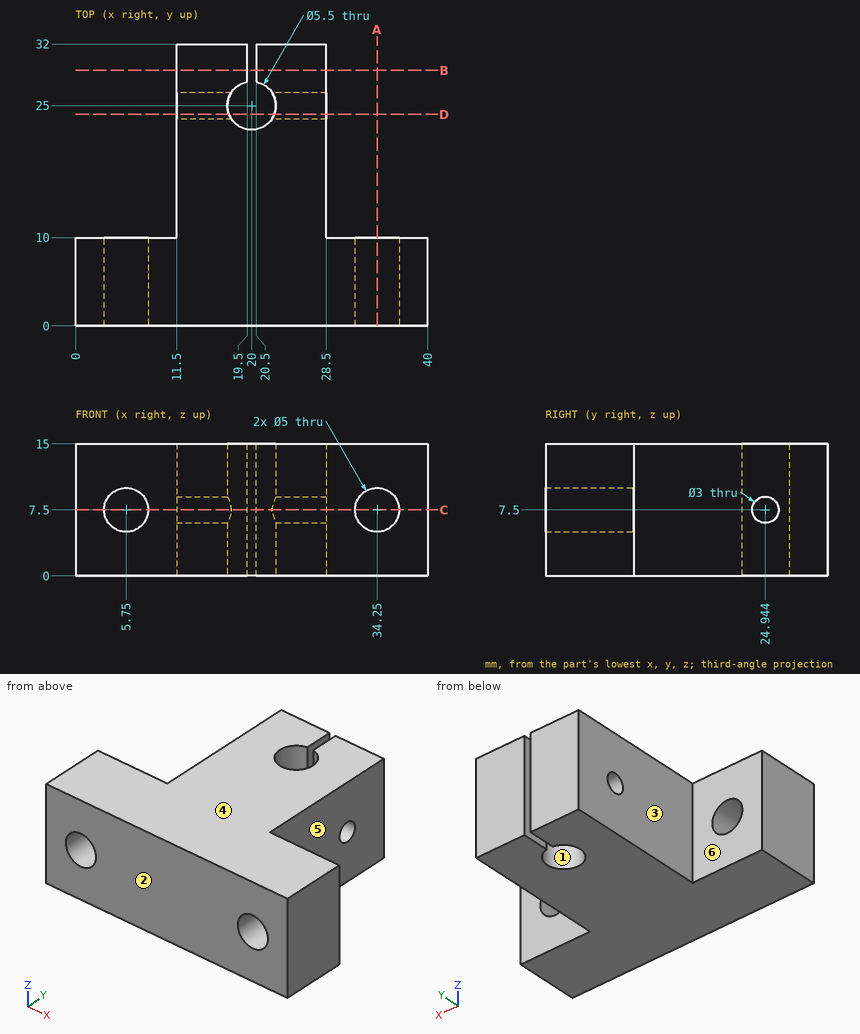
Could you check a few things on this drawing? It's one solid part, dimensions in mm from its lowest x, y, z. A direction names the side the tool comes from. Coordinates: 2 decimals unless noted, no trailing zeros. Loops run counter-clockwise (first coordinate to the right, second up) from the corner with the lowest first, then second, coordinate; pieces in that order, holes last.
1. Imagine slicing it at C-C (z = 7.5). Please give me the cut outline in (x, y).
2. Imagine slicing it at A-A (x = 34.25). Please give me the cut outline in (y, z), and give its area (3 significant figures).
3. Imagine slicing it at D-D (y = 24). Please give me the cut outline in (x, z).
4. For P1, Ø4.5, axis at x = 34.25, z = 7.5, coming from the -Y side; P2, Ø2, axis at y = 29.5, z = 7, coming from the -X side; P3, Ø4.5, axis at y = 29, z = 9, coming from the +X side; P4, Ø6, axis at x = 3.5, z = 11, coming from the +Y side, each with a flat end and sliding along its axis, tell me the tip position at first contact or that it passes through.
5. I need wall thicknesses on L1, parallel to X at y = 25, z = 13; L2, parallel to Z at x = 34.25, y = 2.75; L3, parallel to X at y = 30.5, z = 14.5. Which ranges of each line are inside material? Lowest first, please.
6. For the marked faces 4, 5 and 6, which set-ups out of +Z, -Z, +X, -X, +Y, -Y let a thin tool reach every point of the face, with its end or its side?
7. Imagine slicing it at B-B (y = 29). Please give me the cut outline in (x, z).
8. We'd pull the mould along X, two halves only. Please class the marked faces 1, 2 and 3: released by +X, released by -X, zero draft, split by the parting line, or undercut.
Computed values:
1. outline: (0, 0) - (3.25, 0) - (3.25, 10) - (0, 10) - close; (8.25, 0) - (31.75, 0) - (31.75, 10) - (28.5, 10) - (28.5, 23.44) - (22.27, 23.44) arc R2.75 cw to (17.73, 23.44) - (11.5, 23.44) - (11.5, 10) - (8.25, 10) - close; (11.5, 26.44) - (17.66, 26.44) arc R2.75 cw to (19.5, 27.7) - (19.5, 32) - (11.5, 32) - close; (20.5, 27.7) arc R2.75 cw to (22.34, 26.44) - (28.5, 26.44) - (28.5, 32) - (20.5, 32) - close; (36.75, 0) - (40, 0) - (40, 10) - (36.75, 10) - close
2. outline: (0, 0) - (10, 0) - (10, 5) - (0, 5) - close; (0, 10) - (10, 10) - (10, 15) - (0, 15) - close
2. area: 100 mm2
3. outline: (11.5, 0) - (17.44, 0) - (17.44, 6.33) - (11.5, 6.33) - close; (11.5, 8.67) - (17.44, 8.67) - (17.44, 15) - (11.5, 15) - close; (22.56, 0) - (28.5, 0) - (28.5, 6.33) - (22.56, 6.33) - close; (22.56, 8.67) - (28.5, 8.67) - (28.5, 15) - (22.56, 15) - close
4. P1: passes through
4. P2: stops at x = 11.5
4. P3: stops at x = 28.5
4. P4: stops at y = 10
5. L1: x = 11.5 to 17.25, 22.75 to 28.5
5. L2: z = 0 to 5, 10 to 15
5. L3: x = 11.5 to 19.5, 20.5 to 28.5
6. face 4: +Z, +X, -X, +Y, -Y
6. face 5: +Z, -Z, +X, +Y
6. face 6: +Z, -Z, -X, +Y
7. outline: (11.5, 0) - (19.5, 0) - (19.5, 15) - (11.5, 15) - close; (20.5, 0) - (28.5, 0) - (28.5, 15) - (20.5, 15) - close
8. face 1: undercut
8. face 2: zero draft
8. face 3: released by -X
